Work out the finished part from the listing and answer in its coordinate system (mm). A direction names the side the tool comes from. Round coordinates to 2 decimals unless told otherwise and drop trailing zeros. Order: outer loops, then holes, each group sorted by start corner. A loop starts at its lowest first (then second) coordinate and runs counter-clockwise, first axis right, second up. Notation, with made-up numbers: (-32, 48) - (-23, 48) arc R15 ccw to (-23, 60) - close; hole circle Ø5 at (67.25, -20). An arc over 180 degrees is marked (long way). One line per question, with ' | ' between items. Start each with the question number.
from build123d import *

# Parameters (mm, degrees)
BOSS_EXTRU_1_DEPTH           = 30
ESQUISSE2_W                  = 110
ESQUISSE2_H                  = 15
ENL_V_MAT_EXTRU_1_DEPTH      = 30
ENL_V_START                  = -10
ESQUISSE3_W                  = 44.19
ESQUISSE3_H                  = 7.5
ENL_V_MAT_EXTRU_2_DEPTH      = 10
ESQUISSE4_W                  = 5
ESQUISSE4_H                  = 7.5
BOSS_EXTRU_2_DEPTH           = 10
ESQUISSE5_W                  = 7.5
ESQUISSE5_H                  = 3
BOSS_EXTRU_3_DEPTH           = 6
ESQUISSE6_W                  = 7.5
ESQUISSE6_H                  = 3
BOSS_EXTRU_4_DEPTH           = 5.5
CONG_1_R                     = 10
ESQUISSE7_W                  = 110
ESQUISSE7_H                  = 7.5
BOSS_EXTRU_5_DEPTH           = 10
ENL_V_MAT_EXTRU_3_DEPTH      = 72.632743909
ENL_V_MAT_EXTRU_3_DEPTH_BACK = 72.632743909
ESQUISSE8_R                  = 1.5
CONG_2_R                     = 15
CONG_3_R                     = 15
CONG_4_R                     = 15
CONG_5_R                     = 15
CONG_6_R                     = 10


with BuildPart() as part:
    # Esquisse1 → Boss.-Extru.1 (new body)
    with BuildSketch(Plane.XY):
        with BuildLine():
            Line((-55, 10), (55, 10))
            ThreePointArc((55, 10), (65, 0), (55, -10))
            Line((55, -10), (-55, -10))
            ThreePointArc((-55, -10), (-65, 0), (-55, 10))
        make_face()
        with BuildLine():
            Line((-55, 1.5), (55, 1.5))
            ThreePointArc((55, 1.5), (56.5, 0), (55, -1.5))
            Line((55, -1.5), (-55, -1.5))
            ThreePointArc((-55, -1.5), (-56.5, 0), (-55, 1.5))
        make_face(mode=Mode.SUBTRACT)
    extrude(amount=BOSS_EXTRU_1_DEPTH)

    # Esquisse2 → Enlèv. mat.-Extru.1 (cut)
    with BuildSketch(Plane(origin=(0, 10, 0), x_dir=(1, 0, 0), z_dir=(0, 1, 0))):
        with Locations((0, -15)):
            Rectangle(ESQUISSE2_W, ESQUISSE2_H)
    extrude(amount=-ENL_V_MAT_EXTRU_1_DEPTH, mode=Mode.SUBTRACT)

    # Esquisse3 → Enlèv. mat.-Extru.2 (cut)
    with BuildSketch(Plane(origin=(0, 10, 0), x_dir=(1, 0, 0), z_dir=(0, 1, 0)).offset(ENL_V_START)):
        with Locations((0, -26.25)):
            Rectangle(ESQUISSE3_W, ESQUISSE3_H)
    extrude(amount=-ENL_V_MAT_EXTRU_2_DEPTH, mode=Mode.SUBTRACT)

    # Esquisse4 → Boss.-Extru.2 (add)
    with BuildSketch(Plane(origin=(0, -1.5, 0), x_dir=(1, 0, 0), z_dir=(0, 1, 0))):
        with Locations((-24.595, -26.25)):
            Rectangle(ESQUISSE4_W, ESQUISSE4_H)
        with Locations((24.595, -26.25)):
            Rectangle(ESQUISSE4_W, ESQUISSE4_H)
    extrude(amount=BOSS_EXTRU_2_DEPTH)

    # Esquisse5 → Boss.-Extru.3 (add)
    with BuildSketch(Plane(origin=(27.095, 0, 0), x_dir=(0, 0, -1), z_dir=(1, 0, 0))):
        with Locations((-26.25, 0)):
            Rectangle(ESQUISSE5_W, ESQUISSE5_H)
    extrude(amount=BOSS_EXTRU_3_DEPTH)

    # Esquisse6 → Boss.-Extru.4 (add)
    with BuildSketch(Plane.ZY.offset(27.095)):
        with Locations((26.25, 0)):
            Rectangle(ESQUISSE6_W, ESQUISSE6_H)
    extrude(amount=BOSS_EXTRU_4_DEPTH)

    # Congé1
    cong_1_edges = [part.edges().sort_by_distance(p)[0] for p in [
        (22.095, -10, 26.25),
        (-22.095, -10, 26.25),
    ]]
    fillet(cong_1_edges, radius=CONG_1_R)

    # Esquisse7 → Boss.-Extru.5 (add)
    with BuildSketch(Plane(origin=(0, 10, 0), x_dir=(1, 0, 0), z_dir=(0, 1, 0))):
        with Locations((0, -3.75)):
            Rectangle(ESQUISSE7_W, ESQUISSE7_H)
        with Locations((0, -26.25)):
            Rectangle(ESQUISSE7_W, ESQUISSE7_H)
    extrude(amount=BOSS_EXTRU_5_DEPTH)

    # Esquisse8 → Enlèv. mat.-Extru.3 (cut, two sides: drawn at the far end of the back side and taken through both)
    with BuildSketch(Plane.XY.offset(7.5).offset(-ENL_V_MAT_EXTRU_3_DEPTH_BACK)):
        with Locations((-35, 15)):
            Circle(ESQUISSE8_R)
        with Locations((35, 15)):
            Circle(ESQUISSE8_R)
    extrude(amount=ENL_V_MAT_EXTRU_3_DEPTH + ENL_V_MAT_EXTRU_3_DEPTH_BACK, mode=Mode.SUBTRACT)

    # Congé2
    cong_2_edges = [part.edges().sort_by_distance(p)[0] for p in [
        (-55, 10, 3.75),
    ]]
    fillet(cong_2_edges, radius=CONG_2_R - 0.0001)  # a hair under: the kernel refuses the full size

    # Congé3
    cong_3_edges = [part.edges().sort_by_distance(p)[0] for p in [
        (55, 10, 3.75),
    ]]
    fillet(cong_3_edges, radius=CONG_3_R - 0.0001)  # a hair under: the kernel refuses the full size

    # Congé4
    cong_4_edges = [part.edges().sort_by_distance(p)[0] for p in [
        (-55, 10, 26.25),
    ]]
    fillet(cong_4_edges, radius=CONG_4_R - 0.0001)  # a hair under: the kernel refuses the full size

    # Congé5
    cong_5_edges = [part.edges().sort_by_distance(p)[0] for p in [
        (55, 10, 26.25),
    ]]
    fillet(cong_5_edges, radius=CONG_5_R - 0.0001)  # a hair under: the kernel refuses the full size

    # Congé6
    cong_6_edges = [part.edges().sort_by_distance(p)[0] for p in [
        (-55, 20, 3.75),
        (55, 20, 3.75),
        (55, 20, 26.25),
        (-55, 20, 26.25),
    ]]
    fillet(cong_6_edges, radius=CONG_6_R)


solid = part.part
1) For faces 1 (the cylindrical face through (24.947, -6.993, 26.197)), 2 (the flat face through (33.095, 0, 26)), 3 (the flat face through (-1, 1.5, 4)), 4 (the flat face through (-55, -6, 15)), determine the directions among +Z, -Z, +X, -X, +Y, -Y from which every point of the face is accessible in a straight line to the end or side of a thin tool.
2) Determine the mould class of faces 5 (the flat face through (-1, 20, 26)), 6 (the cylindrical face through (33.8, 14.1, 26.2)), 7 (the cylindrical face through (-65, 0, 15)) for opening direction X: released by +X, released by -X, zero draft, split by the parting line, or undercut.
3) Straight lines are drawn through the part: line 1 (Y direction, x = 35, z = 28); line 2 (Y direction, x = 22.5, z = 7); line 3 (Z direction, x = -7, y = 4). For each, find the intervals that lie inside material, in ascending order.
4) Flat-ended cylindrical pins translate along their axes: pin 1 (0.9 mm diameter, centred on y = -0.5, z = 25.5, fed in from +X); pin 2 (1.8 mm diameter, centred on x = -35, y = 15, fed in from -Z); pin 3 (12 mm diameter, centred on y = 13, z = 15, fed in from -X); pin 4 (3 mm diameter, centred on y = 14, z = 4, fed in from +X). Find the tip coordinate at first contact, or state that the pin passes through.
5) Section A-A on z = 13 is taken. Give the vertices of the cut face in (x, y), and give its area (3 significant figures).
6) Section B-B on x = 35 is taken. Give the vertices of the cut face in (y, z).
7) Section C-C on x = -41 is taken. Give the vertices of the cut face in (y, z), and give its area (3 significant figures).
8) Section D-D on x = 3 is taken. Give the vertices of the cut face in (y, z).
Recorded:
1) face 1: +Z, -Y | face 2: +Z, -Z | face 3: -Z | face 4: +Y, -Y
2) face 5: zero draft | face 6: undercut | face 7: released by -X
3) line 1: y = -10 to -1.5, 1.5 to 13.5, 16.5 to 20 | line 2: y = -10 to -1.5, 1.5 to 20 | line 3: z = 0 to 7.5, 22.5 to 30
4) pin 1: stops at x = 65 | pin 2: passes through | pin 3: stops at x = -62.14 | pin 4: stops at x = 57.01
5) outline: (-55, -10) - (-55, -1.5) arc R1.5 cw to (-55, 1.5) - (-55, 10) arc R10 ccw to start; (55, -10) arc R10 ccw to (55, 10) - (55, 1.5) arc R1.5 cw to (55, -1.5) - close | area: 307 mm²
6) outline: (-10, 0) - (-1.5, 0) - (-1.5, 7.5) - (-10, 7.5) - close; (-10, 22.5) - (-1.5, 22.5) - (-1.5, 30) - (-10, 30) - close; (1.5, 0) - (13.5, 0) - (13.5, 7.5) - (1.5, 7.5) - close; (1.5, 22.5) - (13.5, 22.5) - (13.5, 30) - (1.5, 30) - close; (16.5, 0) - (20, 0) - (20, 7.5) - (16.5, 7.5) - close; (16.5, 22.5) - (20, 22.5) - (20, 30) - (16.5, 30) - close
7) outline: (-10, 0) - (-1.5, 0) - (-1.5, 7.5) - (-10, 7.5) - close; (-10, 22.5) - (-1.5, 22.5) - (-1.5, 30) - (-10, 30) - close; (1.5, 0) - (20, 0) - (20, 7.5) - (1.5, 7.5) - close; (1.5, 22.5) - (20, 22.5) - (20, 30) - (1.5, 30) - close | area: 405 mm²
8) outline: (-10, 0) - (-1.5, 0) - (-1.5, 7.5) - (-10, 7.5) - close; (1.5, 0) - (20, 0) - (20, 7.5) - (1.5, 7.5) - close; (1.5, 22.5) - (20, 22.5) - (20, 30) - (1.5, 30) - close
